from build123d import *

# Parameters (mm, degrees)
SKETCH1_R                      = 10
BOSS_EXTRUDE1_DEPTH            = 10
SKETCH4_R                      = 15
BOSS_EXTRUDE4_DEPTH            = 5
BOSS_EXTRUDE2_DEPTH            = 10
SKETCH3_W                      = 10
SKETCH3_H                      = 10
BOSS_EXTRUDE3_DEPTH            = 232
M5_CLEARANCE_HOLE1_D           = 5.5
M5_CLEARANCE_HOLE1_CSINK_D     = 5.55
M5_CLEARANCE_HOLE1_CSINK_ANGLE = 90
M5_CLEARANCE_HOLE2_D           = 5.5
M5_CLEARANCE_HOLE2_CSINK_D     = 5.55
M5_CLEARANCE_HOLE2_CSINK_ANGLE = 90


with BuildPart() as part:
    # Sketch1 → Boss-Extrude1 (new body)
    with BuildSketch(Plane(origin=(0, 0, 0), x_dir=(1, 0, 0), z_dir=(0, 1, 0))):
        with Locations(Location((0, 0, 0), (0, 0, 270))):
            Circle(SKETCH1_R)
    extrude(amount=BOSS_EXTRUDE1_DEPTH)

    # Sketch4 → Boss-Extrude4 (add)
    with BuildSketch(Plane(origin=(0, 10, 0), x_dir=(1, 0, 0), z_dir=(0, 1, 0))):
        with Locations(Location((0, 0, 0), (0, 0, 270))):
            Circle(SKETCH4_R)
    extrude(amount=BOSS_EXTRUDE4_DEPTH)

    # Sketch2 → Boss-Extrude2 (add)
    with BuildSketch(Plane(origin=(0, 15, 0), x_dir=(1, 0, 0), z_dir=(0, 1, 0))):
        with BuildLine():
            Line((-25, 50), (-25, 5))
            Line((-25, 5), (-14.142135624, 5))
            ThreePointArc((-14.142135624, 5), (0, 15), (14.142135624, 5))
            Line((14.142135624, 5), (25, 5))
            Line((25, 5), (25, 50))
            Line((25, 50), (-25, 50))
        make_face()
        with BuildLine():
            Line((-14.142135624, 5), (-25, 5))
            Line((-25, 5), (-100, 5))
            Line((-100, 5), (-100, -5))
            Line((-100, -5), (-25, -5))
            Line((-25, -5), (-14.142135624, -5))
            ThreePointArc((-14.142135624, -5), (-15, 0), (-14.142135624, 5))
        make_face()
        with BuildLine():
            ThreePointArc((14.142135624, -5), (0, -15), (-14.142135624, -5))
            Line((-14.142135624, -5), (-25, -5))
            Line((-25, -5), (-25, -50))
            Line((-25, -50), (25, -50))
            Line((25, -50), (25, -5))
            Line((25, -5), (14.142135624, -5))
        make_face()
        with BuildLine():
            Line((25, 5), (14.142135624, 5))
            ThreePointArc((14.142135624, 5), (14.783978395, 2.536529681), (15, 0))
            ThreePointArc((15, 0), (14.783978395, -2.536529681), (14.142135624, -5))
            Line((14.142135624, -5), (25, -5))
            Line((25, -5), (100, -5))
            Line((100, -5), (100, 5))
            Line((100, 5), (25, 5))
        make_face()
        with BuildLine():
            Line((14.142135624, 5), (-14.142135624, 5))
            ThreePointArc((-14.142135624, 5), (-15, 0), (-14.142135624, -5))
            Line((-14.142135624, -5), (14.142135624, -5))
            ThreePointArc((14.142135624, -5), (14.783978395, -2.536529681), (15, 0))
            ThreePointArc((15, 0), (14.783978395, 2.536529681), (14.142135624, 5))
        make_face()
        with BuildLine():
            ThreePointArc((14.142135624, 5), (0, 15), (-14.142135624, 5))
            Line((-14.142135624, 5), (14.142135624, 5))
        make_face()
        with BuildLine():
            Line((14.142135624, -5), (-14.142135624, -5))
            ThreePointArc((-14.142135624, -5), (0, -15), (14.142135624, -5))
        make_face()
    extrude(amount=BOSS_EXTRUDE2_DEPTH)

    # Sketch3 → Boss-Extrude3 (add)
    with BuildSketch(Plane(origin=(0, 25, 0), x_dir=(1, 0, 0), z_dir=(0, 1, 0))):
        with Locations((-95, 0)):
            Rectangle(SKETCH3_W, SKETCH3_H)
        with Locations((95, 0)):
            Rectangle(SKETCH3_W, SKETCH3_H)
    extrude(amount=BOSS_EXTRUDE3_DEPTH)

    # M5 Clearance Hole1 (through all)
    with Locations(Plane.ZY.offset(100)):
        with Locations((0, 252)):
            CounterSinkHole(M5_CLEARANCE_HOLE1_D / 2, M5_CLEARANCE_HOLE1_CSINK_D / 2, counter_sink_angle=M5_CLEARANCE_HOLE1_CSINK_ANGLE)

    # M5 Clearance Hole2 (through all)
    with Locations(Plane(origin=(0, 25, 0), x_dir=(1, 0, 0), z_dir=(0, 1, 0))):
        with Locations((-20, 0), (20, 0)):
            CounterSinkHole(M5_CLEARANCE_HOLE2_D / 2, M5_CLEARANCE_HOLE2_CSINK_D / 2, counter_sink_angle=M5_CLEARANCE_HOLE2_CSINK_ANGLE)


solid = part.part
Here's how the part is built. I have some questions about the finished solid (model axes, mm). A direction names the side the tool comes from. Round coordinates to 2 decimals unless told otherwise and drop trailing zeros. Loops run counter-clockwise (first coordinate to the right, second up) from the corner with the lowest first, then second, coordinate; pieces in that order, holes last.
1. If we section it at A-A on x = 20: Write out the boundary of the cut face in (y, z) (3 decimals).
Answer list:
outline: (15, -50) - (25, -50) - (25, -2.775) - (24.975, -2.75) - (15, -2.75) - close; (15, 2.75) - (24.975, 2.75) - (25, 2.775) - (25, 50) - (15, 50) - close
2. We'd pull the mould along Z, two halves only. Please class faces 1 (the face through (95.07, 249.315, 0.596)), 2 (the face through (-15.3, 15, -0.2)), 3 (the face through (-94.918, 249.315, 0.596)), 4 (the face through (0, 20, 50)): +Z half, -Z half, draft (parallel to the pull), parting line (faces both ways), or undercut.
Answer list:
face 1: undercut
face 2: draft
face 3: undercut
face 4: +Z half
3. If I drill on line 1 along Y through (x, z) = (96.25, 0); line 2 along Z through (x, y) = (-95, 252); line 3 along X through (y, z) = (101, 2), over which ranges is the centre line in solid material (lowest first)?
Answer list:
line 1: y = 15 to 249.25, 254.75 to 257
line 2: z = -5 to -2.75, 2.75 to 5
line 3: x = -100 to -90, 90 to 100
4. Which directions (+Z, -Z, +X, -X, +Y, -Y) give clear straight access to the entire face, cutting with the end or side of a thin tool? Please do faces 5 (the face through (-90.5, 117.5, -5)), 6 (the face through (-9.76, 4.93, -2.17)), 7 (the face through (25, 20, -27)), 8 (the face through (-25, 20, 27)), 9 (the face through (25, 20, 28)).
Answer list:
face 5: -Z, -X, +Y, -Y
face 6: -Y
face 7: -Z, +X, +Y, -Y
face 8: +Z, -X, +Y, -Y
face 9: +Z, +X, +Y, -Y
5. If we section it at C-C on y = 152.5: Write out the boundary of the cut face in (x, z), plus the area to 3 significant figures.
Answer list:
outline: (-100, -5) - (-90, -5) - (-90, 5) - (-100, 5) - close; (90, -5) - (100, -5) - (100, 5) - (90, 5) - close
area: 200 mm2
6. If we section it at D-D on x = 0: Write out the boundary of the cut face in (y, z).
Answer list:
outline: (0, -10) - (10, -10) - (10, -15) - (15, -15) - (15, -50) - (25, -50) - (25, 50) - (15, 50) - (15, 15) - (10, 15) - (10, 10) - (0, 10) - close
7. If we section it at B-B on y = 252: Write out the boundary of the cut face in (x, z) (3 decimals).
Answer list:
outline: (-100, -5) - (-90, -5) - (-90, -2.75) - (-99.975, -2.75) - (-100, -2.775) - close; (-100, 2.775) - (-99.975, 2.75) - (-90, 2.75) - (-90, 5) - (-100, 5) - close; (90, -5) - (100, -5) - (100, -2.75) - (90, -2.75) - close; (90, 2.75) - (100, 2.75) - (100, 5) - (90, 5) - close
8. For P1, Ø11, axis at y = 21, z = 28.5, coming from the -X side; P2, Ø11, axis at y = 21.5, z = 18, coming from the +X side; P3, Ø9, axis at x = 20, z = 0, coming from the +Y side; P4, Ø6.5, axis at y = 252, z = 0, coming from the -X side, each with a flat end and sliding along its axis, tell me the tip position at first contact or that it passes through.
Answer list:
P1: stops at x = -25
P2: stops at x = 25
P3: stops at y = 25
P4: stops at x = -100
